Autodesk Inventor part; units mm, degrees
ref_plane "YZ Plane" through (0, 0, 0) normal (1, 0, 0) x (0, 1, 0)
ref_plane "XZ Plane" through (0, 0, 0) normal (0, 1, 0) x (-1, 0, 0)
ref_plane "XY Plane" through (0, 0, 0) normal (0, 0, 1) x (1, 0, 0)
sketch "Sketch1" plane through (0, 0, 0) normal (0, 0, 1) x (1, 0, 0)
  line L0 (0, 0) -> (12.7, 0)
  line L1 (12.7, 0) -> (12.7, 12.7)
  line L2 (12.7, 12.7) -> (0, 12.7)
  line L3 (0, 12.7) -> (0, 0)
  dimension "d0" = 12.7
  dimension "d1" = 12.7
extrude "Extrusion1" add sketch "Sketch1" along normal blind 6.35
sketch "Sketch2" plane through (0, 0, 6.35) normal (0, 0, 1) x (1, 0, 0)
  line L0 (0, 12.7) -> (0, 0) construction
  line L1 (0, 0) -> (12.7, 0) construction
  line L2 (0, 12.7) -> (12.7, 0) construction
  line L3 (12.7, 12.7) -> (0, 12.7) construction
  line L4 (0, 0) -> (12.7, 12.7) construction
  point P0 (6.35, 6.35)
hole "Hole1" at (6.35, 6.35, 6.35) direction (0, 0, -1) diameter 6.35 end through all counterbore diameter 10.16 counterbore depth 4.1275
chamfer "Chamfer1" distance 1.27 angle 45 4 edges at (12.7, 6.35, 0) (6.35, 12.7, 0) (0, 6.35, 0) (6.35, 0, 0)
fillet "Fillet1" radius 3.175 4 edges at (12.7, 12.7, 3.81) (12.7, 0, 3.81) (0, 12.7, 3.81) (0, 0, 3.81)
properties part number "testswitch"
Geometry check sheet. Reference: the model listing, model coordinates, mm. A direction names the side the tool comes from. Coordinates: 2 decimals unless noted, no trailing zeros. Order: outer loops, then holes, each group sorted by start corner. A loop starts at its lowest first (then second) coordinate and runs counter-clockwise, first axis right, second up. Notation, with made-up numbers: (50.25, 7) - (94.25, 7) arc R23 ccw to (94.25, 30) - close; hole circle Ø6 at (34, 43). An arc over 180 degrees is marked (long way). Answer in a Markdown table with one row per item. Add a question column.
1. Section check D-D (x = 10.25). Enter the section's corners in (y, z).
2. Access from +Z, -Z, +X, -X, +Y, -Y to the whole of each face (thin tool, end or side, straight path). Record for faces 1 (the face through (8.3, 1.66, 4.26)), 2 (the face through (6, 12.7, 4)).
3. Draft check along X on faces 3 (the face through (9.45, 7.04, 1.1)), 4 (the face through (11.75, 0.91, 3.39)), 5 (the face through (0, 6, 4)). Enter one of: +X half, -X half, draft (parallel to the pull), parting line (faces both ways), or undercut.
4. Material ranges on L1, parallel to Y at x = 6.35, z = 3.55; L2, parallel to X at y = 6.35, z = 1.5 (3 decimals), recorded low to high. Write a range as [from, to].
5. Section check C-C (z = 3.25). Enter the section's corners in (x, y) (3 decimals).
6. Gauge pin test, flat ends, axial feed: pin 1 Ø1 at (y, z) = (10, 5.5) entering from +X; pin 2 Ø1 at (x, y) = (6, 8) entering from -Z; pin 3 Ø5 at (x, y) = (5.5, 5.5) entering from +Z. Record the tip position at first contact, or that the pin passes through.
Data:
| question | item | result |
|---|---|---|
| 1 | outline | (0.08, 1.19) - (1.27, 0) - (11.43, 0) - (12.62, 1.19) - (12.62, 6.35) - (9.61, 6.35) - (9.61, 2.22) - (3.09, 2.22) - (3.09, 6.35) - (0.08, 6.35) - close |
| 2 | face 1 | +Z |
| 2 | face 2 | +Z, -Z, +X, -X, +Y |
| 3 | face 3 | undercut |
| 3 | face 4 | +X half |
| 3 | face 5 | -X half |
| 4 | L1 | y = [0, 1.27], [11.43, 12.7] |
| 4 | L2 | x = [0, 3.175], [9.525, 12.7] |
| 5 | outline | (0, 3.175) arc R3.175 ccw to (3.175, 0) - (9.525, 0) arc R3.175 ccw to (12.7, 3.175) - (12.7, 9.525) arc R3.175 ccw to (9.525, 12.7) - (3.175, 12.7) arc R3.175 ccw to (0, 9.525) - close; hole circle Ø10.16 at (6.35, 6.35) |
| 6 | pin 1 | stops at x = 12.7 |
| 6 | pin 2 | passes through |
| 6 | pin 3 | stops at z = 2.22 |
